Could you check a few things on this model? Use its own coordinates, in mm. A direction names the side the tool comes from. Give positions to 0.01 mm unless a question says otherwise; leave off trailing zeros. Loops run counter-clockwise (first coordinate to the right, second up) from the corner with the lowest first, then second, coordinate; pieces in that order, holes last. Notation, with made-up numbers: M 83,34.5 L 111,34.5 A25 ccw 111,69.5 Z; hole C 68,2 d6. An arc over 180 degrees is marked long. Return JSON: item names as keys, results as strings. Group by question number.
1. If we section it at D-D (z = 11): Write out the boundary of the cut face in (x, y) (3 decimals), plus the area to 3 significant figures.
2. If we mould it in two halves opening along X, with no side actions, what happens to faces 6 (the flat face through (-152.4, 6, -1)), 7 (the flat face through (161, -2.794, -1)), 8 (the cylindrical face through (158.315, -0.039, 35.954))? For each: +X half, -X half, draft (parallel to the pull), parting line (faces both ways), or undercut.
3. For pin 1 (4 mm diameter, centred on y = 5, z = -35.5, fed in from +X); pin 2 (5 mm diameter, centred on x = 160.655, z = 38.1, fed in from +Y); pin 3 (5.5 mm diameter, centred on y = 6.5, z = -12.5, fed in from -X); pin 4 (8.5 mm diameter, centred on x = -160.5, z = 17, fed in from +Y), each with a flat end and sliding along its axis, tell me the tip position at first contact or that it passes through.
4. If we section it at A-A (z = 38.1): Write out the boundary of the cut face in (x, y) (3 decimals), plus the area to 3 significant figures.
5. If we section it at B-B (y = -6.25): Write out the boundary of the cut face in (x, z).
6. For faces 1 (the flat face through (-152.4, -6, -1)), 2 (the flat face through (152.4, -6, 1)), 3 (the flat face through (161, 2.794, -1)), 4 (the flat face through (-2, 9.525, 16)), 5 (the flat face through (-161, 2.794, -1)), which set-ups out of +Z, -Z, +X, -X, +Y, -Y let a thin tool reach every point of the face, with its end or its side?
7. If we section it at C-C (z = -46.99): Write out the boundary of the cut face in (x, y) (3 decimals).
8. Please list where these lines run through material, in increasing order: line 1 (Z direction, x = 114.3, y = -0.75); line 2 (X direction, y = 8.75, z = -33); line 3 (X direction, y = -7, z = 40).
```python
from build123d import *

# Parameters (mm, degrees)
BOSS_EXTRUDE1_DEPTH         = 9.525
F_8_32_TAPPED_HOLE1_D       = 3.4544
SKETCH6_W                   = 16.51
SKETCH6_H                   = 152.4
BOSS_EXTRUDE2_DEPTH         = 2.794
F_1_4_0_25_DIAMETER_HOLE1_D = 6.35


with BuildPart() as part:
    # Sketch1 → Boss-Extrude1 (new, symmetric)
    with BuildSketch(Plane(origin=(0, 0, 0), x_dir=(1, 0, 0), z_dir=(0, 1, 0))):
        with BuildLine():
            ThreePointArc((0, 7.62), (-61.289836841, 26.369500976), (-101.6, 76.2))
            Line((-101.6, 76.2), (-152.4, 76.2))
            Line((-152.4, 76.2), (-152.4, -76.2))
            Line((-152.4, -76.2), (152.4, -76.2))
            Line((152.4, -76.2), (152.4, 76.2))
            Line((152.4, 76.2), (101.6, 76.2))
            ThreePointArc((101.6, 76.2), (61.289836841, 26.369500976), (0, 7.62))
        make_face()
    extrude(amount=BOSS_EXTRUDE1_DEPTH, both=True)

    # #8-32 Tapped Hole1 (through all)
    with Locations(Plane(origin=(0, 9.525, 0), x_dir=(1, 0, 0), z_dir=(0, 1, 0))):
        with Locations((-139.7, -19.05), (-114.3, -19.05), (-63.5, -19.05)):
            f_8_32_tapped_hole1 = Hole(F_8_32_TAPPED_HOLE1_D / 2)

    # Mirror1: #8-32 Tapped Hole1 across plane
    add(f_8_32_tapped_hole1.mirror(Plane(origin=(0, 0, 0), x_dir=(0, 0, 1), z_dir=(1, 0, 0))), mode=Mode.SUBTRACT)

    # Sketch6 → Boss-Extrude2 (add, symmetric)
    with BuildSketch(Plane(origin=(0, 0, 0), x_dir=(1, 0, 0), z_dir=(0, 1, 0))):
        with Locations((-160.655, 0)):
            Rectangle(SKETCH6_W, SKETCH6_H)
    boss_extrude2 = extrude(amount=BOSS_EXTRUDE2_DEPTH, both=True)

    # 1/4 (0.25) Diameter Hole1 (through all)
    with Locations(Plane(origin=(0, 2.794, 0), x_dir=(1, 0, 0), z_dir=(0, 1, 0))):
        with Locations((-160.655, 46.99), (-160.655, -38.1)):
            f_1_4_0_25_diameter_hole1 = Hole(F_1_4_0_25_DIAMETER_HOLE1_D / 2)

    # Mirror2: Boss-Extrude2, 1/4 (0.25) Diameter Hole1 across plane
    add(boss_extrude2.mirror(Plane(origin=(0, 0, 0), x_dir=(0, 0, 1), z_dir=(1, 0, 0))))
    add(f_1_4_0_25_diameter_hole1.mirror(Plane(origin=(0, 0, 0), x_dir=(0, 0, 1), z_dir=(1, 0, 0))), mode=Mode.SUBTRACT)


solid = part.part
```
Answer:
{
 "1": {"outline": "M -168.91,-2.794 L -152.4,-2.794 L -152.4,-9.525 L 152.4,-9.525 L 152.4,-2.794 L 168.91,-2.794 L 168.91,2.794 L 152.4,2.794 L 152.4,9.525 L -152.4,9.525 L -152.4,2.794 L -168.91,2.794 Z", "area": "5,990 mm²"},
 "2": {"face 6": "-X half", "face 7": "draft", "face 8": "undercut"},
 "3": {"pin 1": "stops at x = 152.4", "pin 2": "passes through", "pin 3": "stops at x = -152.4", "pin 4": "stops at y = 2.79"},
 "4": {"outline": "M -168.91,-2.794 L -163.83,-2.794 L -163.83,2.794 L -168.91,2.794 Z; M -157.48,-2.794 L -152.4,-2.794 L -152.4,-9.525 L 152.4,-9.525 L 152.4,-2.794 L 157.48,-2.794 L 157.48,2.794 L 152.4,2.794 L 152.4,9.525 L -152.4,9.525 L -152.4,2.794 L -157.48,2.794 Z; M 163.83,-2.794 L 168.91,-2.794 L 168.91,2.794 L 163.83,2.794 Z", "area": "5,920 mm²"},
 "5": {"outline": "M -152.4,-76.2 L -101.6,-76.2 A109.55 cw 101.6,-76.2 L 152.4,-76.2 L 152.4,76.2 L -152.4,76.2 Z; hole C -139.7,19.05 d3.45; hole C -114.3,19.05 d3.45; hole C -63.5,19.05 d3.45; hole C 63.5,19.05 d3.45; hole C 114.3,19.05 d3.45; hole C 139.7,19.05 d3.45"},
 "6": {"face 1": "+Z, -Z, -X, -Y", "face 2": "+Z, -Z, +X, -Y", "face 3": "+Z, -Z, +X, +Y", "face 4": "+Z, -Z, +X, -X, +Y", "face 5": "+Z, -Z, -X, +Y"},
 "7": {"outline": "M -168.91,-2.794 L -163.83,-2.794 L -163.83,2.794 L -168.91,2.794 Z; M -157.48,-2.794 L -152.4,-2.794 L -152.4,-9.525 L -84.118,-9.525 L -84.118,9.525 L -152.4,9.525 L -152.4,2.794 L -157.48,2.794 Z; M 84.118,-9.525 L 152.4,-9.525 L 152.4,-2.794 L 157.48,-2.794 L 157.48,2.794 L 152.4,2.794 L 152.4,9.525 L 84.118,9.525 Z; M 163.83,-2.794 L 168.91,-2.794 L 168.91,2.794 L 163.83,2.794 Z"},
 "8": {"line 1": "z = -76.2 to 17.32, 20.78 to 76.2", "line 2": "x = -152.4 to -70.12, 70.12 to 152.4", "line 3": "x = -152.4 to 152.4"}
}
